Could you check a few things on this model? Use its own coordinates, in mm. Face numbers are marked on the shaded views. A direction names the side the tool comes from. Coordinates: 2 decimals unless noted, no trailing zeros. Loops run counter-clockwise (first coordinate to the right, second up) from the corner with the lowest first, then second, coordinate; pieces in that order, holes last.
1) Will these pins go through, and if not, where does the flat tip stop? P1, Ø1.6, axis at x = 0.5, z = 1.5, coming from the -Y side; P2, Ø1.5, axis at x = -52.5, z = 3.5, coming from the +Y side; P3, Ø2, axis at y = 39, z = 1.5, coming from the -X side.
2) Imagine slicing it at A-A on x = 0. Please give me the cut outline in (y, z) (3 decimals), plus the area to 3 significant figures.
3) Imagine slicing it at C-C on z = 1.15. Give the number of separate pieces and of enclosed holes in the cut face, plus the area to 3 significant figures.
4) Thinking about a two-plate mould opening in Y: for the marked faces 3 and 4, which applies, released by +Y, released by -Y, zero draft, split by the parting line, or undercut?
5) For the marked faces 1 and 2, which set-ups out of +Z, -Z, +X, -X, +Y, -Y let a thin tool reach every point of the face, with its end or its side?
6) If I drill on line 1 along X through (y, z) = (1, 2.6); line 2 along Y through (x, z) = (0, 2.05); line 3 along X through (y, z) = (-48, 1.95), over which ranges is the centre line in solid material (lowest first)?
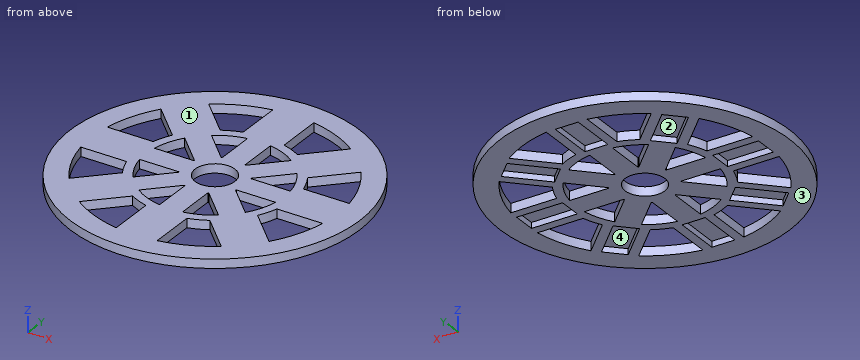
```python
from build123d import *

# Parameters (mm, degrees)
SKETCH1_R           = 80
SKETCH1_R_2         = 11
SKETCH1_W           = 12.7
SKETCH1_H           = 25.4
SKETCH1_W_2         = 25.4
SKETCH1_H_2         = 12.7
BOSS_EXTRUDE1_DEPTH = 5
SKETCH1_3_W         = 25.4
SKETCH1_3_H         = 12.7
SKETCH1_3_W_2       = 12.7
SKETCH1_3_H_2       = 25.4
CUT_EXTRUDE2_DEPTH  = 3.175
CUT_EXTRUDE3_DEPTH  = 19
CUT_EXTRUDE4_DEPTH  = 19


with BuildPart() as part:
    # Sketch1 → Boss-Extrude1 (new body)
    # profile 1 of 9: a face of its own
    with BuildSketch(Plane.XY):
        Circle(SKETCH1_R)
        Circle(SKETCH1_R_2, mode=Mode.SUBTRACT)
        Polygon((33.905770158, 24.925514037), (51.8662824, 42.886026279), (42.886026279, 51.8662824), (24.925514037, 33.905770158), align=None, mode=Mode.SUBTRACT)
        with Locations((0, 54.3)):
            Rectangle(SKETCH1_W, SKETCH1_H, mode=Mode.SUBTRACT)
        Polygon((-24.925514037, 33.905770158), (-42.886026279, 51.8662824), (-51.8662824, 42.886026279), (-33.905770158, 24.925514037), align=None, mode=Mode.SUBTRACT)
        with Locations((-54.3, 0)):
            Rectangle(SKETCH1_W_2, SKETCH1_H_2, mode=Mode.SUBTRACT)
        Polygon((-33.905770158, -24.925514037), (-51.8662824, -42.886026279), (-42.886026279, -51.8662824), (-24.925514037, -33.905770158), align=None, mode=Mode.SUBTRACT)
        with Locations((0, -54.3)):
            Rectangle(SKETCH1_W, SKETCH1_H, mode=Mode.SUBTRACT)
        Polygon((24.925514037, -33.905770158), (42.886026279, -51.8662824), (51.8662824, -42.886026279), (33.905770158, -24.925514037), align=None, mode=Mode.SUBTRACT)
        with Locations((54.3, 0)):
            Rectangle(SKETCH1_W_2, SKETCH1_H_2, mode=Mode.SUBTRACT)
    # profile 2 of 9: a face of its own
    with BuildSketch(Plane.XY):
        with Locations((-54.3, 0)):
            Rectangle(SKETCH1_W_2, SKETCH1_H_2)
    # profile 3 of 9: a face of its own
    with BuildSketch(Plane.XY):
        Polygon((-24.925514037, 33.905770158), (-33.905770158, 24.925514037), (-51.8662824, 42.886026279), (-42.886026279, 51.8662824), align=None)
    # profile 4 of 9: a face of its own
    with BuildSketch(Plane.XY):
        with Locations((0, 54.3)):
            Rectangle(SKETCH1_W, SKETCH1_H)
    # profile 5 of 9: a face of its own
    with BuildSketch(Plane.XY):
        Polygon((33.905770158, 24.925514037), (24.925514037, 33.905770158), (42.886026279, 51.8662824), (51.8662824, 42.886026279), align=None)
    # profile 6 of 9: a face of its own
    with BuildSketch(Plane.XY):
        with Locations((54.3, 0)):
            Rectangle(SKETCH1_W_2, SKETCH1_H_2)
    # profile 7 of 9: a face of its own
    with BuildSketch(Plane.XY):
        Polygon((24.925514037, -33.905770158), (33.905770158, -24.925514037), (51.8662824, -42.886026279), (42.886026279, -51.8662824), align=None)
    # profile 8 of 9: a face of its own
    with BuildSketch(Plane.XY):
        with Locations((0, -54.3)):
            Rectangle(SKETCH1_W, SKETCH1_H)
    # profile 9 of 9: a face of its own
    with BuildSketch(Plane.XY):
        Polygon((-33.905770158, -24.925514037), (-24.925514037, -33.905770158), (-42.886026279, -51.8662824), (-51.8662824, -42.886026279), align=None)
    extrude(amount=BOSS_EXTRUDE1_DEPTH)

    # Sketch1_3 → Cut-Extrude2 (cut)
    with BuildSketch(Plane.XY):
        Polygon((33.905770158, -24.925514037), (51.8662824, -42.886026279), (42.886026279, -51.8662824), (24.925514037, -33.905770158), align=None)
        with Locations((54.3, 0)):
            Rectangle(SKETCH1_3_W, SKETCH1_3_H)
        with Locations((0, -54.3)):
            Rectangle(SKETCH1_3_W_2, SKETCH1_3_H_2)
        Polygon((-24.925514037, -33.905770158), (-42.886026279, -51.8662824), (-51.8662824, -42.886026279), (-33.905770158, -24.925514037), align=None)
        with Locations((-54.3, 0)):
            Rectangle(SKETCH1_3_W, SKETCH1_3_H)
        Polygon((-33.905770158, 24.925514037), (-51.8662824, 42.886026279), (-42.886026279, 51.8662824), (-24.925514037, 33.905770158), align=None)
        with Locations((0, 54.3)):
            Rectangle(SKETCH1_3_W_2, SKETCH1_3_H_2)
        Polygon((24.925514037, 33.905770158), (42.886026279, 51.8662824), (51.8662824, 42.886026279), (33.905770158, 24.925514037), align=None)
    extrude(amount=CUT_EXTRUDE2_DEPTH, mode=Mode.SUBTRACT)

    # Sketch2 → Cut-Extrude3 (cut)
    with BuildSketch(Plane(origin=(0, 0, 0), x_dir=(-1, 0, 0), z_dir=(0, 0, -1))):
        with BuildLine():
            ThreePointArc((31.116508001, -22.13625188), (35.280233052, -14.613551014), (37.655387628, -6.35))
            Line((37.655387628, -6.35), (15.911210185, -6.35))
            ThreePointArc((15.911210185, -6.35), (15.827464249, -6.55595035), (15.741052679, -6.760796558))
            Line((15.741052679, -6.760796558), (31.116508001, -22.13625188))
        make_face()
        with BuildLine():
            Line((15.911210185, 6.35), (37.655387628, 6.35))
            ThreePointArc((37.655387628, 6.35), (35.280233052, 14.613551014), (31.116508001, 22.13625188))
            Line((31.116508001, 22.13625188), (15.741052679, 6.760796558))
            ThreePointArc((15.741052679, 6.760796558), (15.827464249, 6.55595035), (15.911210185, 6.35))
        make_face()
        with BuildLine():
            Line((6.760796558, 15.741052679), (22.13625188, 31.116508001))
            ThreePointArc((22.13625188, 31.116508001), (14.613551014, 35.280233052), (6.35, 37.655387628))
            Line((6.35, 37.655387628), (6.35, 15.911210185))
            ThreePointArc((6.35, 15.911210185), (6.55595035, 15.827464249), (6.760796558, 15.741052679))
        make_face()
        with BuildLine():
            Line((-6.35, 15.911210185), (-6.35, 37.655387628))
            ThreePointArc((-6.35, 37.655387628), (-14.613551014, 35.280233052), (-22.13625188, 31.116508001))
            Line((-22.13625188, 31.116508001), (-6.760796558, 15.741052679))
            ThreePointArc((-6.760796558, 15.741052679), (-6.55595035, 15.827464249), (-6.35, 15.911210185))
        make_face()
        with BuildLine():
            ThreePointArc((-31.116508001, 22.13625188), (-35.280233052, 14.613551014), (-37.655387628, 6.35))
            Line((-37.655387628, 6.35), (-15.911210185, 6.35))
            ThreePointArc((-15.911210185, 6.35), (-15.827464249, 6.55595035), (-15.741052679, 6.760796558))
            Line((-15.741052679, 6.760796558), (-31.116508001, 22.13625188))
        make_face()
        with BuildLine():
            ThreePointArc((-37.655387628, -6.35), (-35.280233052, -14.613551014), (-31.116508001, -22.13625188))
            Line((-31.116508001, -22.13625188), (-15.741052679, -6.760796558))
            ThreePointArc((-15.741052679, -6.760796558), (-15.827464249, -6.55595035), (-15.911210185, -6.35))
            Line((-15.911210185, -6.35), (-37.655387628, -6.35))
        make_face()
        with BuildLine():
            ThreePointArc((-22.13625188, -31.116508001), (-14.613551014, -35.280233052), (-6.35, -37.655387628))
            Line((-6.35, -37.655387628), (-6.35, -15.911210185))
            ThreePointArc((-6.35, -15.911210185), (-6.55595035, -15.827464249), (-6.760796558, -15.741052679))
            Line((-6.760796558, -15.741052679), (-22.13625188, -31.116508001))
        make_face()
        with BuildLine():
            ThreePointArc((6.35, -37.655387628), (14.613551014, -35.280233052), (22.13625188, -31.116508001))
            Line((22.13625188, -31.116508001), (6.760796558, -15.741052679))
            ThreePointArc((6.760796558, -15.741052679), (6.55595035, -15.827464249), (6.35, -15.911210185))
            Line((6.35, -15.911210185), (6.35, -37.655387628))
        make_face()
    extrude(amount=-CUT_EXTRUDE3_DEPTH, mode=Mode.SUBTRACT)

    # Sketch3 → Cut-Extrude4 (cut)
    with BuildSketch(Plane(origin=(0, 0, 0), x_dir=(-1, 0, 0), z_dir=(0, 0, -1))):
        with BuildLine():
            Line((-21.389980131, -37.441304064), (-39.350492373, -55.401816306))
            ThreePointArc((-39.350492373, -55.401816306), (-26.005085041, -62.781828996), (-11.35, -67))
            Line((-11.35, -67), (-11.35, -41.6))
            ThreePointArc((-11.35, -41.6), (-16.501523042, -39.838200729), (-21.389980131, -37.441304064))
        make_face()
        with BuildLine():
            Line((-41.6, -11.35), (-67, -11.35))
            ThreePointArc((-67, -11.35), (-62.781828996, -26.005085041), (-55.401816306, -39.350492373))
            Line((-55.401816306, -39.350492373), (-37.441304064, -21.389980131))
            ThreePointArc((-37.441304064, -21.389980131), (-39.838200729, -16.501523042), (-41.6, -11.35))
        make_face()
        with BuildLine():
            Line((-37.441304064, 21.389980131), (-55.401816306, 39.350492373))
            ThreePointArc((-55.401816306, 39.350492373), (-62.781828996, 26.005085041), (-67, 11.35))
            Line((-67, 11.35), (-41.6, 11.35))
            ThreePointArc((-41.6, 11.35), (-39.838200729, 16.501523042), (-37.441304064, 21.389980131))
        make_face()
        with BuildLine():
            Line((-11.35, 41.6), (-11.35, 67))
            ThreePointArc((-11.35, 67), (-26.005085041, 62.781828996), (-39.350492373, 55.401816306))
            Line((-39.350492373, 55.401816306), (-21.389980131, 37.441304064))
            ThreePointArc((-21.389980131, 37.441304064), (-16.501523042, 39.838200729), (-11.35, 41.6))
        make_face()
        with BuildLine():
            Line((21.389980131, 37.441304064), (39.350492373, 55.401816306))
            ThreePointArc((39.350492373, 55.401816306), (26.005085041, 62.781828996), (11.35, 67))
            Line((11.35, 67), (11.35, 41.6))
            ThreePointArc((11.35, 41.6), (16.501523042, 39.838200729), (21.389980131, 37.441304064))
        make_face()
        with BuildLine():
            Line((41.6, 11.35), (67, 11.35))
            ThreePointArc((67, 11.35), (62.781828996, 26.005085041), (55.401816306, 39.350492373))
            Line((55.401816306, 39.350492373), (37.441304064, 21.389980131))
            ThreePointArc((37.441304064, 21.389980131), (39.838200729, 16.501523042), (41.6, 11.35))
        make_face()
        with BuildLine():
            Line((37.441304064, -21.389980131), (55.401816306, -39.350492373))
            ThreePointArc((55.401816306, -39.350492373), (62.781828996, -26.005085041), (67, -11.35))
            Line((67, -11.35), (41.6, -11.35))
            ThreePointArc((41.6, -11.35), (39.838200729, -16.501523042), (37.441304064, -21.389980131))
        make_face()
        with BuildLine():
            Line((11.35, -41.6), (11.35, -67))
            ThreePointArc((11.35, -67), (26.005085041, -62.781828996), (39.350492373, -55.401816306))
            Line((39.350492373, -55.401816306), (21.389980131, -37.441304064))
            ThreePointArc((21.389980131, -37.441304064), (16.501523042, -39.838200729), (11.35, -41.6))
        make_face()
    extrude(amount=-CUT_EXTRUDE4_DEPTH, mode=Mode.SUBTRACT)


solid = part.part
```
Filled in:
1. P1: stops at y = -80
1. P2: stops at y = 61.01
1. P3: stops at x = -70.4
2. outline: (-80, 0) - (-67, 0) - (-67, 3.175) - (-41.6, 3.175) - (-41.6, 0) - (-11, 0) - (-11, 5) - (-80, 5) - close; (11, 0) - (41.6, 0) - (41.6, 3.175) - (67, 3.175) - (67, 0) - (80, 0) - (80, 5) - (11, 5) - close
2. area: 529 mm2
3. separate pieces: 1
3. enclosed holes: 25
3. area: 11,500 mm2
4. face 3: zero draft
4. face 4: undercut
5. face 1: +Z, +X, -X, +Y, -Y
5. face 2: -Z
6. line 1: x = -79.99 to -67, -41.6 to -10.95, 10.95 to 41.6, 67 to 79.99
6. line 2: y = -80 to -67, -41.6 to -11, 11 to 41.6, 67 to 80
6. line 3: x = -64 to -46.75, -39.02 to -31.95, -11.35 to -6.35, 6.35 to 11.35, 31.95 to 39.02, 46.75 to 64
